Here's how the part is built. I have some questions about the finished solid (model axes, mm). A direction names the side the tool comes from. Round coordinates to 2 decimals unless told otherwise and drop trailing zeros. Loops run counter-clockwise (first coordinate to the right, second up) from the corner with the lowest first, then second, coordinate; pieces in that order, holes last. Notation, with made-up numbers: (36.5, -3.5) -> (54.5, -3.5) arc R25 cw to (54.5, 34.5) -> close; hole circle Ø1 at (79, 5.25). An arc over 180 degrees is marked (long way). One line per item, written item: value. Start each with the question number.
```python
from build123d import *

# Parameters (mm, degrees)
M2_SCREW_CLIP_BODY_PROFILE_W       = 7
M2_SCREW_CLIP_BODY_PROFILE_H       = 3.5
M2_SCREW_CLIP_BODY_PROFILE_R       = 1.15
M2_SCREW_CLIP_BODY_DEPTH           = 5.8
BOARD_START                        = 3.9
BOARD_EDGE_RETAINING_TOE_PROFILE_W = 7
BOARD_EDGE_RETAINING_TOE_PROFILE_H = 1.3
BOARD_EDGE_RETAINING_TOE_DEPTH     = 1.9


with BuildPart() as part:
    # M2 screw clip body profile → M2 screw clip body (new body)
    with BuildSketch(Plane.XY):
        with Locations((0, 0.05)):
            Rectangle(M2_SCREW_CLIP_BODY_PROFILE_W, M2_SCREW_CLIP_BODY_PROFILE_H)
        Circle(M2_SCREW_CLIP_BODY_PROFILE_R, mode=Mode.SUBTRACT)
    extrude(amount=M2_SCREW_CLIP_BODY_DEPTH)

    # Board edge retaining toe profile → Board edge retaining toe (add)
    with BuildSketch(Plane.XY.offset(BOARD_START)):
        with Locations((0, 2.45)):
            Rectangle(BOARD_EDGE_RETAINING_TOE_PROFILE_W, BOARD_EDGE_RETAINING_TOE_PROFILE_H)
    extrude(amount=BOARD_EDGE_RETAINING_TOE_DEPTH)


solid = part.part
```
Q1. I want a section at C-C on z = 2.85. Please give me the cut outline in (x, y).
Q2. Which directions (+Z, -Z, +X, -X, +Y, -Y) give clear straight access to the entire face, cutting with the end or side of a thin tool? Please do faces 1 (the flat face through (0, 1.3, 5.8)), 2 (the flat face through (0, 1.8, 2)).
Q3. Will this pin go through, and if not, where does the flat tip stop? P1, Ø1, axis at x = -1, z = 1, coming from the +Y side.
Q4. If we mould it in two halves opening along X, with no side actions, what happens to faces 3 (the flat face through (3.5, 0, 3)), 4 (the cylindrical face through (-0.91, -0.7, 2.86)), 5 (the flat face through (0, -1.7, 3))? For each: released by +X, released by -X, zero draft, split by the parting line, or undercut.
Q5. If I drill on line 1 along Y through (x, z) = (0, 3.6); line 2 along Y through (x, z) = (2.75, 3); line 3 along Y through (x, z) = (0, 4.5), over which ranges is the centre line in solid material (lowest first)?
Q6. I want a section at A-A on y = 0. Please give me the cut outline in (x, z).
Q7. I want a section at B-B on x = 0. Please give me the cut outline in (y, z), plus the area to 3 significant figures.
Q8. I want a section at D-D on y = -0.8. Please give me the cut outline in (x, z), plus the area to 3 significant figures.
Answers below:
1. outline: (-3.5, -1.7) -> (3.5, -1.7) -> (3.5, 1.8) -> (-3.5, 1.8) -> close; hole circle Ø2.3 at (0, 0)
2. face 1: +Z, +X, -X, +Y, -Y
2. face 2: -Z, +X, -X, +Y
3. P1: stops at y = 1.8
4. face 3: released by +X
4. face 4: undercut
4. face 5: zero draft
5. line 1: y = -1.7 to -1.15, 1.15 to 1.8
5. line 2: y = -1.7 to 1.8
5. line 3: y = -1.7 to -1.15, 1.15 to 3.1
6. outline: (-3.5, 0) -> (-1.15, 0) -> (-1.15, 5.8) -> (-3.5, 5.8) -> close; (1.15, 0) -> (3.5, 0) -> (3.5, 5.8) -> (1.15, 5.8) -> close
7. outline: (-1.7, 0) -> (-1.15, 0) -> (-1.15, 5.8) -> (-1.7, 5.8) -> close; (1.15, 0) -> (1.8, 0) -> (1.8, 3.9) -> (3.1, 3.9) -> (3.1, 5.8) -> (1.15, 5.8) -> close
7. area: 9.43 mm^2
8. outline: (-3.5, 0) -> (-0.83, 0) -> (-0.83, 5.8) -> (-3.5, 5.8) -> close; (0.83, 0) -> (3.5, 0) -> (3.5, 5.8) -> (0.83, 5.8) -> close
8. area: 31.0 mm^2
